Here's the drawing with two shaded views (mm, measured from the low corner). I have some questions. A direction names the side the tool comes from. Coordinates: 2 decimals unless noted, no trailing zeros. Write each loop counter-clockwise with the first axis right and the second up, starting at its lowest first coordinate (ties: lowest second). Pieces come first, ordered by that corner, then holes.
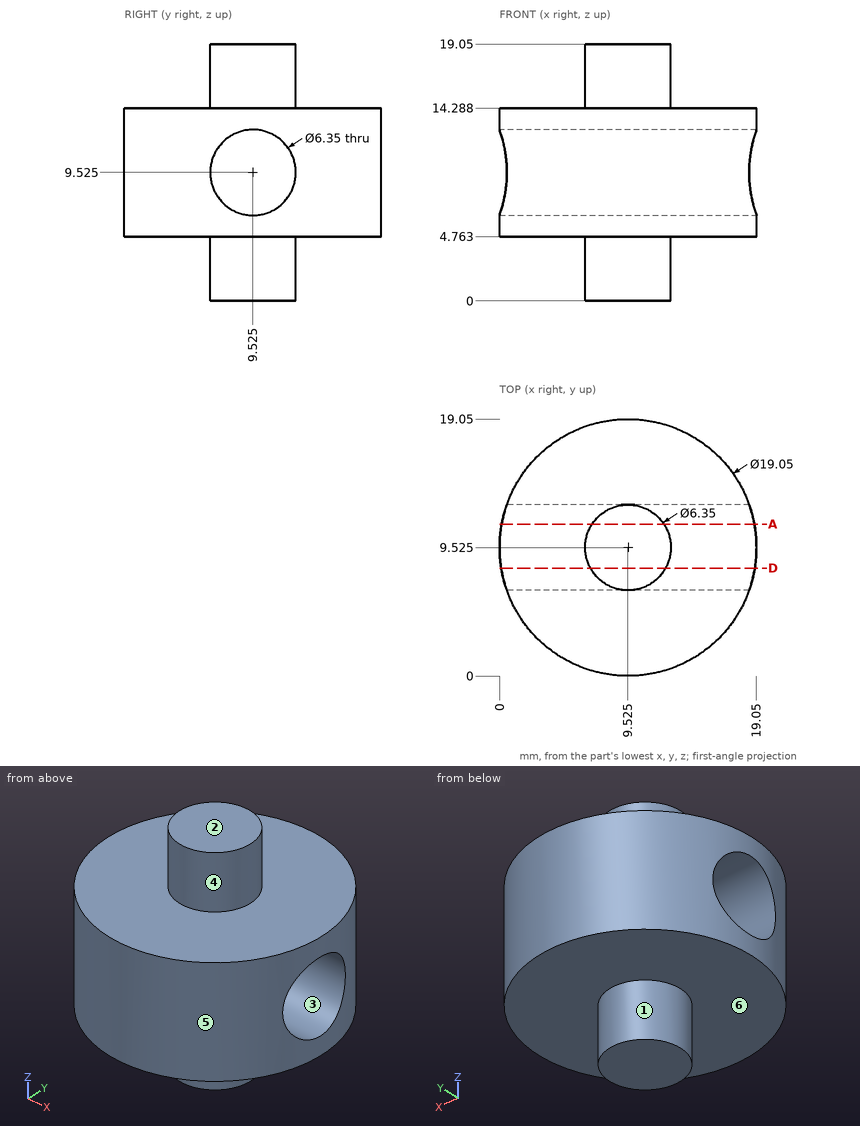
1. For pin 1 (4 mm diameter, centred on x = 5, z = 5.5, fed in from +Y); pin 2 (2 mm diameter, centred on x = 7, z = 15.5, fed in from +Y); pin 3 (4 mm diameter, centred on x = 6, y = 15.5, fed in from -Z), each with a flat end and sliding along its axis, tell me the tip position at first contact or that it passes through.
Verdict:
pin 1: stops at y = 18.71
pin 2: stops at y = 12.31
pin 3: stops at z = 4.76
2. I want a section at D-D on y = 8. Please give me the cut outline in (x, z).
Verdict:
outline: (0.12, 4.76) - (6.74, 4.76) - (6.74, 0) - (12.31, 0) - (12.31, 4.76) - (18.93, 4.76) - (18.93, 6.74) - (0.12, 6.74) - close; (0.12, 12.31) - (18.93, 12.31) - (18.93, 14.29) - (12.31, 14.29) - (12.31, 19.05) - (6.74, 19.05) - (6.74, 14.29) - (0.12, 14.29) - close
3. If we mould it in two halves opening along Y, with no side actions, what happens to the marked faces 1, 2 and 3? For each: pulls with the +Y half, pulls with the -Y half, needs draft (parallel to the pull), parting line crosses it, or undercut.
Verdict:
face 1: parting line crosses it
face 2: needs draft
face 3: undercut
4. On a 3-axis mill with a long thin cutter (end or side, diameter ignored), from which of +Z, -Z, +X, -X, +Y, -Y can I reach the whole of each face in a straight line? I mean the marked faces 4, 5 and 6. Say none if no direction works.
Verdict:
face 4: +Z
face 5: +Z, -Z
face 6: -Z
5. Please list where these lines run through material, in increasing order: line 1 along Y through (x, z) = (13, 11.5) (1 decimal); line 2 along Y through (x, z) = (17, 12) (1 decimal); line 3 along Z through (x, y) = (15.5, 10.25) (1 decimal).
Verdict:
line 1: y = 0.7 to 7, 12 to 18.4
line 2: y = 3.6 to 7.5, 11.5 to 15.4
line 3: z = 4.8 to 6.4, 12.6 to 14.3
6. I want a section at A-A on y = 11.25. Please give me the cut outline in (x, z), plus the area to 3 significant figures.
Verdict:
outline: (0.16, 4.76) - (6.86, 4.76) - (6.86, 0) - (12.19, 0) - (12.19, 4.76) - (18.89, 4.76) - (18.89, 6.86) - (0.16, 6.86) - close; (0.16, 12.19) - (18.89, 12.19) - (18.89, 14.29) - (12.19, 14.29) - (12.19, 19.05) - (6.86, 19.05) - (6.86, 14.29) - (0.16, 14.29) - close
area: 129 mm2
